```python
from build123d import *

# Parameters (mm, degrees)
SKETCH026_R                = 2.875
SKETCH026_R_2              = 1.55
EXTRUDE026_DEPTH           = 15
EXTRUDE026_PLACEMENT_ANGLE = 270
SKETCH025_R                = 1.55
EXTRUDE025_DEPTH           = 4
EXTRUDE025_PLACEMENT_ANGLE = 270
FILLET029_R                = 1


with BuildPart() as spacer001:
    # Sketch026 → Extrude026 (new body)
    with BuildSketch(Plane.YZ):
        with Locations((3, 38.75)):
            Circle(SKETCH026_R)
        with Locations((3, 38.75)):
            Circle(SKETCH026_R_2, mode=Mode.SUBTRACT)
        with Locations((3, 3)):
            Circle(SKETCH026_R)
        with Locations((3, 3)):
            Circle(SKETCH026_R_2, mode=Mode.SUBTRACT)
        with Locations((103.75, 3)):
            Circle(SKETCH026_R)
        with Locations((103.75, 3)):
            Circle(SKETCH026_R_2, mode=Mode.SUBTRACT)
        with Locations((103.75, 38.75)):
            Circle(SKETCH026_R)
        with Locations((103.75, 38.75)):
            Circle(SKETCH026_R_2, mode=Mode.SUBTRACT)
    extrude(amount=EXTRUDE026_DEPTH)


with BuildPart() as spacer001_1:
    # Extrude026 placement: moved
    add(spacer001.part.moved(Location((0, -2, 0))).rotate(Axis((0, -2, 0), (0, 0, 1)), EXTRUDE026_PLACEMENT_ANGLE))


with BuildPart() as top_fillet001:
    # Sketch025 → Extrude025 (new body)
    with BuildSketch(Plane.YZ):
        Polygon((106.25, 0), (106.25, 41.75), (0, 41.75), (0, 0), (18.25, 0), (18.25, 15), (88, 15), (88, 0), align=None)
        with Locations((3, 3)):
            Circle(SKETCH025_R, mode=Mode.SUBTRACT)
        with Locations((3, 38.75)):
            Circle(SKETCH025_R, mode=Mode.SUBTRACT)
        with Locations((103.75, 38.75)):
            Circle(SKETCH025_R, mode=Mode.SUBTRACT)
        with Locations((103.75, 3)):
            Circle(SKETCH025_R, mode=Mode.SUBTRACT)
    extrude(amount=EXTRUDE025_DEPTH)


with BuildPart() as top_fillet001_1:
    # Extrude025 placement: moved
    add(top_fillet001.part.moved(Location((0, -17, 0))).rotate(Axis((0, -17, 0), (0, 0, 1)), EXTRUDE025_PLACEMENT_ANGLE))

    # Fusion029: union spacer001
    add(spacer001_1.part)

    # Fillet029
    fillet029_edges = [top_fillet001_1.edges().sort_by_distance(p)[0] for p in [
        (106.25, -19, 0),
        (106.25, -19, 41.75),
        (88, -19, 0),
        (0, -19, 41.75),
        (88, -19, 15),
        (0, -19, 0),
        (18.25, -19, 15),
        (18.25, -19, 0),
    ]]
    fillet(fillet029_edges, radius=FILLET029_R)


solid = top_fillet001_1.part
```
CAD build for the part. Positions are in the model's coordinates, mm. A direction names the side the tool comes from. Give positions to 0.01 mm unless a question says otherwise; leave off trailing zeros. Loops run counter-clockwise (first coordinate to the right, second up) from the corner with the lowest first, then second, coordinate; pieces in that order, holes last. Notation, with made-up numbers: M 48,86.5 L 90,86.5 A10 cw 90,103.5 Z; hole C -3,43.5 d9. An arc over 180 degrees is marked long. Use one line per item in the form item = value.
Item 1: Flat gauge pins, fed straight in: pin 1 (1.9 mm diameter, centred on x = 3, z = 3, fed in from +Y); pin 2 (3 mm diameter, centred on x = 49, y = -18.5, fed in from -Z); pin 3 (2 mm diameter, centred on y = -18, z = 16, fed in from +X). Where does each tip first touch, or does it go through?
Determined:
pin_1 = through
pin_2 = 15
pin_3 = 106.25
Item 2: Slice it at B-B (y = -15). List the corners of the cut face in (x, z) (3 decimals).
Determined:
outline = C 3,3 d5.75; C 3,38.75 d5.75; C 103.75,3 d5.75; C 103.75,38.75 d5.75; hole C 3,3 d3.1; hole C 3,38.75 d3.1; hole C 103.75,3 d3.1; hole C 103.75,38.75 d3.1
Item 3: Slice it at D-D (z = 8). List the corners of the cut face in (x, y).
Determined:
outline = M 0,-21 L 18.25,-21 L 18.25,-17 L 0,-17 Z; M 88,-21 L 106.25,-21 L 106.25,-17 L 88,-17 Z
Item 4: Two-plate mould, pull along X, no slides. Class faces 4 (the face through (4.55, -9.4, 41.17)), 5 (the face through (9, -19, 0)), 6 (the face through (106.25, -19, 21)): pulls with the +X half, pulls with the -X half, needs draft (parallel to the pull), parting line crosses it, or undercut.
Determined:
face_4 = undercut
face_5 = needs draft
face_6 = pulls with the +X half
Item 5: Which spindle directions (+Z, -Z, +X, -X, +Y, -Y) get a long thin tool onto all of the face, cutting with end or side? Do faces 1 (the face through (18.25, -19, 7)), 2 (the face through (106.492, -9.395, 3.864)), 3 (the face through (54, -19, 41.75)). Say none if no direction does.
Determined:
face_1 = -Z, +Y, -Y
face_2 = +Y
face_3 = +Z, +X, -X, +Y, -Y
Item 6: Drill centre lines: probe 1 along Z at (x, y) = (103.75, -8.25) (3 decimals); probe 2 along X at (y, z) = (-9, 39); probe 3 along X at (y, z) = (-6.75, 37.5). Where is each one in solid material? Low to high. Write a range as from..to.
Determined:
probe_1 = 0.125..1.45, 4.55..5.875, 35.875..37.2, 40.3..41.625
probe_2 = 0.14..1.47, 4.53..5.86, 100.89..102.22, 105.28..106.61
probe_3 = 0.41..2.08, 3.92..5.59, 101.16..102.83, 104.67..106.34
Item 7: Slice it at A-A (x = 3). List the corners of the cut face in (y, z) (3 decimals).
Determined:
outline = M -21,0 L -17,0 L -17,0.125 L -2,0.125 L -2,1.45 L -21,1.45 Z; M -21,4.55 L -2,4.55 L -2,5.875 L -17,5.875 L -17,35.875 L -2,35.875 L -2,37.2 L -21,37.2 Z; M -21,40.3 L -2,40.3 L -2,41.625 L -17,41.625 L -17,41.75 L -21,41.75 Z
Item 8: Slice it at C-C (z = 3). List the corners of the cut face in (x, y) (3 decimals).
Determined:
outline = M 0,-21 L 1.45,-21 L 1.45,-2 L 0.125,-2 L 0.125,-17 L 0,-17 Z; M 4.55,-21 L 18.25,-21 L 18.25,-17 L 5.875,-17 L 5.875,-2 L 4.55,-2 Z; M 88,-21 L 102.2,-21 L 102.2,-2 L 100.875,-2 L 100.875,-17 L 88,-17 Z; M 105.3,-21 L 106.25,-21 L 106.25,-17 L 106.625,-17 L 106.625,-2 L 105.3,-2 Z
